from build123d import *

# Parameters (mm, degrees)
BOSS_EXTRUDE1_DEPTH = 23.622
SKETCH5_R           = 1.3843
CUT_EXTRUDE1_DEPTH  = 29.405286863
FILLET1_R           = 0.396875
FILLET2_R           = 0.1984375


with BuildPart() as part:
    # Sketch3 → Boss-Extrude1 (new, symmetric)
    with BuildSketch(Plane.XY):
        Polygon((-6.376363514, 1.397), (-6.376363514, 0.889), (-2.921, 0.889), (-2.921, -1.905), (-10.3124, -1.905), (-10.3124, -5.969), (10.3124, -5.969), (10.3124, -1.905), (2.921, -1.905), (2.921, 0.889), (6.376363514, 0.889), (6.376363514, 1.397), (2.54, 5.969), (-2.54, 5.969), align=None)
    extrude(amount=BOSS_EXTRUDE1_DEPTH, both=True)

    # Sketch5 → Cut-Extrude1 (cut, through all)
    with BuildSketch(Plane.XZ.offset(5.969)):
        with Locations(Location((0, 12.7, 0), (0, 0, 270))):
            Circle(SKETCH5_R)
        with Locations(Location((0, -12.7, 0), (0, 0, 270))):
            Circle(SKETCH5_R)
    extrude(amount=-CUT_EXTRUDE1_DEPTH, mode=Mode.SUBTRACT)

    # Fillet1
    fillet1_edges = [part.edges().sort_by_distance(p)[0] for p in [
        (2.921, 0.889, 0),
        (2.921, -1.905, 0),
        (-2.921, -1.905, 0),
        (-2.921, 0.889, 0),
    ]]
    fillet(fillet1_edges, radius=FILLET1_R)

    # Fillet2
    fillet2_edges = [part.edges().sort_by_distance(p)[0] for p in [
        (-4.847119257, 0.889, 23.622),
        (0, 5.969, -23.622),
        (4.458181757, 3.683, -23.622),
        (6.376363514, 1.143, -23.622),
        (6.8151375, -1.905, -23.622),
        (10.3124, -3.937, -23.622),
        (0, -5.969, -23.622),
        (-10.3124, -3.937, -23.622),
        (-4.847119257, 0.889, -23.622),
        (-6.376363514, 1.143, -23.622),
        (-4.458181757, 3.683, -23.622),
        (-10.3124, -3.937, 23.622),
        (0, -5.969, 23.622),
        (-2.54, 5.969, 0),
        (2.54, 5.969, 0),
        (6.376363514, 1.397, 0),
        (6.376363514, 0.889, 0),
        (10.3124, -1.905, 0),
        (10.3124, -5.969, 0),
        (-10.3124, -5.969, 0),
        (-10.3124, -1.905, 0),
        (-6.376363514, 0.889, 0),
        (-6.376363514, 1.397, 0),
        (10.3124, -3.937, 23.622),
        (6.8151375, -1.905, 23.622),
        (6.376363514, 1.143, 23.622),
        (-4.458181757, 3.683, 23.622),
        (4.458181757, 3.683, 23.622),
        (0, 5.969, 23.622),
        (4.847119257, 0.889, -23.622),
        (4.847119257, 0.889, 23.622),
        (2.921, -0.508, -23.622),
        (2.921, -0.508, 23.622),
        (-2.921, -0.508, -23.622),
        (-2.921, -0.508, 23.622),
        (-6.8151375, -1.905, -23.622),
        (-6.8151375, -1.905, 23.622),
        (3.037241996, 0.772758004, -23.622),
        (3.037241996, 0.772758004, 23.622),
        (-3.037241996, 0.772758004, -23.622),
        (-3.037241996, 0.772758004, 23.622),
        (-3.037241996, -1.788758004, -23.622),
        (-3.037241996, -1.788758004, 23.622),
        (3.037241996, -1.788758004, -23.622),
        (3.037241996, -1.788758004, 23.622),
        (-6.376363514, 1.143, 23.622),
    ]]
    fillet(fillet2_edges, radius=FILLET2_R)


solid = part.part
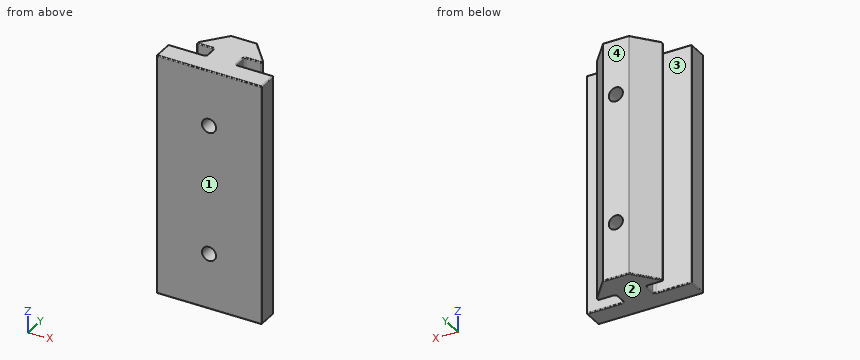
Verification items for the finished model (mm, model axes). Face numbers are marked on the shaded views. Round coordinates to 2 decimals unless told otherwise and drop trailing zeros. Loops run counter-clockwise (first coordinate to the right, second up) from the corner with the lowest first, then second, coordinate; pieces in that order, holes last. Notation, with made-up numbers: (77, -37) - (83, -37) arc R25 ccw to (83, -10) - close; hole circle Ø2 at (-19, 81.25). An arc over 180 degrees is marked (long way). Use a Markdown table: item, result. Add a question column.
1. Release check for a two-part mould opening along Y. For the marked faces 1, 2, 3 and 4 record: released by +Y, released by -Y, zero draft, split by the parting line, or undercut.
2. Gauge pin test, flat ends, axial feed: pin 1 (2 mm diameter, centred on x = 0, z = -12.7, fed in from -Y); pin 2 (1 mm diameter, centred on y = 0, z = 5, fed in from +X); pin 3 (3 mm diameter, centred on y = 1, z = -1.5, fed in from +X); pin 4 (5.5 mm diameter, centred on x = 7, z = 7, fed in from +Y). Record the tip position at first contact, or that the pin passes through.
3. Thickness scan on probe 1 along Y at (x, z) = (-5.5, -6) (3 decimals); probe 2 along Z at (x, y) = (-0.5, -1.5); probe 3 along X at (y, z) = (-2.5, 12.7). Record the ranges inside material, lowest first. Write a range as [from, to].
4. Section check C-C, the plane z = -3. Record the boundary of the cut face in (x, y) (3 decimals), plus the area to 3 significant figures.
5. Section check B-B, the plane x = 0. Record the boundary of the cut face in (y, z).
Checks:
| question | item | result |
|---|---|---|
| 1 | face 1 | released by -Y |
| 1 | face 2 | zero draft |
| 1 | face 3 | undercut |
| 1 | face 4 | released by +Y |
| 2 | pin 1 | passes through |
| 2 | pin 2 | stops at x = 2.92 |
| 2 | pin 3 | stops at x = 6.38 |
| 2 | pin 4 | stops at y = 3.93 |
| 3 | probe 1 | y = [-5.969, -1.905], [0.889, 2.441] |
| 3 | probe 2 | z = [-23.62, -13.99], [-11.41, 11.41], [13.99, 23.62] |
| 3 | probe 3 | x = [-10.31, -1.38], [1.38, 10.31] |
| 4 | outline | (-10.312, -5.771) arc R0.198 ccw to (-10.114, -5.969) - (10.114, -5.969) arc R0.198 ccw to (10.312, -5.771) - (10.312, -2.103) arc R0.198 ccw to (10.114, -1.905) - (3.318, -1.905) arc R0.397 cw to (2.921, -1.508) - (2.921, 0.492) arc R0.397 cw to (3.318, 0.889) - (6.178, 0.889) arc R0.198 ccw to (6.376, 1.087) - (6.376, 1.325) arc R0.198 ccw to (6.33, 1.452) - (2.599, 5.898) arc R0.198 ccw to (2.447, 5.969) - (-2.447, 5.969) arc R0.198 ccw to (-2.599, 5.898) - (-6.33, 1.452) arc R0.198 ccw to (-6.376, 1.325) - (-6.376, 1.087) arc R0.198 ccw to (-6.178, 0.889) - (-3.318, 0.889) arc R0.397 cw to (-2.921, 0.492) - (-2.921, -1.508) arc R0.397 cw to (-3.318, -1.905) - (-10.114, -1.905) arc R0.198 ccw to (-10.312, -2.103) - close |
| 4 | area | 147 mm^2 |
| 5 | outline | (-5.97, -23.42) arc R0.2 ccw to (-5.77, -23.62) - (5.77, -23.62) arc R0.2 ccw to (5.97, -23.42) - (5.97, -14.08) - (-5.97, -14.08) - close; (-5.97, -11.32) - (5.97, -11.32) - (5.97, 11.32) - (-5.97, 11.32) - close; (-5.97, 14.08) - (5.97, 14.08) - (5.97, 23.42) arc R0.2 ccw to (5.77, 23.62) - (-5.77, 23.62) arc R0.2 ccw to (-5.97, 23.42) - close |
